Source: CAD feature listing. Evaluate the final solid. Frame: model axes, mm. A direction names the side the tool comes from. Give positions to 0.01 mm unless a question says otherwise; leave off trailing zeros. Order: outer loops, then holes, each group sorted by start corner. A loop starts at its lowest first (then second) coordinate and runs counter-clockwise, first axis right, second up. Notation, with made-up numbers: M 82,61.5 L 137,61.5 A20 ccw 137,84.5 Z; hole C 67,-6 d1. An arc over 180 degrees is marked long. Answer in a Markdown table with one row per item. Add a question column.
(1) Section query D-D, the plane z = 8. Return loops of the section in (x, y), plus the area to 3 significant figures.
(2) Set-up query: faces 1 (the face through (-1, 6, -4)), 2 (the face through (0.423, 7.222, -8.514)), 3 (the face through (3, 6, -9.5)), 4 (the face through (5.752, 5.387, -0.099)), 5 (the face through (2, 0, 3)). Return all of +Z, -Z, +X, -X, +Y, -Y with unobstructed straight access to the full face (end or side cutting, diameter ignored); none if empty.
(3) Section query A-A, the plane z = 0. Return loops of the section in (x, y).
(4) Pin query (flat end, axial travel): P1, Ø3, axis at x = -5.5, y = 6, coming from the +Z side; P2, Ø2, axis at x = -8, z = 0.5, coming from the +Y side; P3, Ø3, axis at y = 5.5, z = -5.5, coming from the +X side. Return the tip coordinate at first contact, or that it passes through.
(5) Material intervals for line 1 along X through (y, z) = (7, -1.25); line 2 along Z through (x, y) = (1.75, 2.75); line 3 along Y through (x, z) = (8, 1.5), sorted ascending.
(6) Section query C-C, the plane x = 0. Return loops of the section in (y, z).
(7) Mould query, pull axis Z, two halves, no side actions, for faces 6 (the face through (-0.29, 5.39, 5.77)), 7 (the face through (2, 8, 3)), 8 (the face through (-0.406, 3.944, 11.243)). Classes: pulls with the +Z half, pulls with the -Z half, needs draft (parallel to the pull), parting line crosses it, or undercut.
(8) Section query B-B, the plane y = 4. Return loops of the section in (x, z).
from build123d import *

# Parameters (mm, degrees)
BOSS_EXTRU_1_DEPTH                              = 8
SKETCH1_R                                       = 3.2
CUT_EXTRUDE1_DEPTH                              = 18.808003819
ESQUISSE7_W                                     = 7
ESQUISSE7_H                                     = 3.5
ENL_V_MAT_EXTRU_2_DEPTH                         = 18.808003819
CHAMBRAGE_POUR_VIS_T_TE_CYLINDRIQUE_D           = 2.5
CHAMBRAGE_POUR_VIS_T_TE_CYLINDRIQUE_CBORE_D     = 4.5
CHAMBRAGE_POUR_VIS_T_TE_CYLINDRIQUE_CBORE_DEPTH = 5.3
CBORE_FOR_M5_HEX_HEAD_BOLT1_D                   = 4
CBORE_FOR_M5_HEX_HEAD_BOLT1_DEPTH               = 9.499
CBORE_FOR_M5_HEX_HEAD_BOLT1_CBORE_D             = 6.5
CBORE_FOR_M5_HEX_HEAD_BOLT1_CBORE_DEPTH         = 2
CBORE_FOR_M5_HEX_HEAD_BOLT1_TIP                 = 1.201721238


with BuildPart() as part:
    # Esquisse1 → Boss.-Extru.1 (new body)
    with BuildSketch(Plane(origin=(0, 0, 0), x_dir=(1, 0, 0), z_dir=(0, 1, 0))):
        with BuildLine():
            Line((6.025985397, 9.5), (-6.025985397, 9.5))
            ThreePointArc((-6.025985397, 9.5), (0, -11.25), (6.025985397, 9.5))
        make_face()
    extrude(amount=BOSS_EXTRU_1_DEPTH)

    # Sketch1 → Cut-Extrude1 (cut, through all)
    with BuildSketch(Plane(origin=(0, 8, 0), x_dir=(1, 0, 0), z_dir=(0, 1, 0))):
        with Locations(Location((0, 0, 0), (0, 0, 270))):
            Circle(SKETCH1_R)
    extrude(amount=-CUT_EXTRUDE1_DEPTH, mode=Mode.SUBTRACT)

    # Esquisse7 → Enlèv. mat.-Extru.2 (cut, through all)
    with BuildSketch(Plane(origin=(0, 8, 0), x_dir=(1, 0, 0), z_dir=(0, 1, 0))):
        with Locations((0, 5.75)):
            Rectangle(ESQUISSE7_W, ESQUISSE7_H)
    extrude(amount=-ENL_V_MAT_EXTRU_2_DEPTH, mode=Mode.SUBTRACT)

    # Chambrage pour vis à tête cylindrique à 6 pans creux (ou vis CHC) M21 (through all)
    with Locations(Plane(origin=(0, 8, 0), x_dir=(1, 0, 0), z_dir=(0, 1, 0))):
        with Locations((-8, 0), (0, -8), (8, 0)):
            CounterBoreHole(CHAMBRAGE_POUR_VIS_T_TE_CYLINDRIQUE_D / 2, CHAMBRAGE_POUR_VIS_T_TE_CYLINDRIQUE_CBORE_D / 2, CHAMBRAGE_POUR_VIS_T_TE_CYLINDRIQUE_CBORE_DEPTH)

    # CBORE for M5 Hex Head Bolt1
    with Locations(Plane(origin=(0, 0, -9.5), x_dir=(-1, 0, 0), z_dir=(0, 0, -1))):
        with Locations((0, 4)):
            CounterBoreHole(CBORE_FOR_M5_HEX_HEAD_BOLT1_D / 2, CBORE_FOR_M5_HEX_HEAD_BOLT1_CBORE_D / 2, CBORE_FOR_M5_HEX_HEAD_BOLT1_CBORE_DEPTH, depth=CBORE_FOR_M5_HEX_HEAD_BOLT1_DEPTH)
            with Locations((0, 0, -(CBORE_FOR_M5_HEX_HEAD_BOLT1_DEPTH + CBORE_FOR_M5_HEX_HEAD_BOLT1_TIP / 2))):  # 118° drill point
                Cone(0, CBORE_FOR_M5_HEX_HEAD_BOLT1_D / 2, CBORE_FOR_M5_HEX_HEAD_BOLT1_TIP, mode=Mode.SUBTRACT)


solid = part.part
Values follow:
| question | item | result |
|---|---|---|
| 1 | outline | M -7.91,0 L -1.25,0 L -1.25,2.7 L -2.25,2.7 L -2.25,8 L -7.91,8 Z; M 1.25,0 L 7.91,0 L 7.91,8 L 2.25,8 L 2.25,2.7 L 1.25,2.7 Z |
| 1 | area | 96.0 mm² |
| 2 | face 1 | +Y, -Y |
| 2 | face 2 | -Z |
| 2 | face 3 | -Z, +X, -X, +Y, -Y |
| 2 | face 4 | +Y |
| 2 | face 5 | +Z, -Z, +X, -X, -Y |
| 3 | outline | M -11.25,0 L -9.25,0 L -9.25,2.7 L -10.25,2.7 L -10.25,8 L -11.25,8 Z; M -6.75,0 L -3.2,0 L -3.2,8 L -5.75,8 L -5.75,2.7 L -6.75,2.7 Z; M 3.2,0 L 6.75,0 L 6.75,2.7 L 5.75,2.7 L 5.75,8 L 3.2,8 Z; M 9.25,0 L 11.25,0 L 11.25,8 L 10.25,8 L 10.25,2.7 L 9.25,2.7 Z |
| 4 | P1 | stops at z = 10.51 |
| 4 | P2 | stops at y = 2.7 |
| 4 | P3 | stops at x = 10.51 |
| 5 | line 1 | x = -11.18 to -9.87, -6.13 to -2.95, 2.95 to 6.13, 9.87 to 11.18 |
| 5 | line 2 | z = -4 to -2.68, 2.68 to 6.59, 9.41 to 11.11 |
| 5 | line 3 | y = 0 to 2.7 |
| 6 | outline | M 0,-9.5 L 0.75,-9.5 L 0.75,-7.5 L 0,-7.5 Z; M 0,-4 L 2,-4 L 2,-3.2 L 0,-3.2 Z; M 0,3.2 L 8,3.2 L 8,5.75 L 2.7,5.75 L 2.7,6.75 L 0,6.75 Z; M 0,9.25 L 2.7,9.25 L 2.7,10.25 L 8,10.25 L 8,11.25 L 0,11.25 Z; M 6,-4 L 8,-4 L 8,-3.2 L 6,-3.2 Z; M 7.25,-9.5 L 8,-9.5 L 8,-7.5 L 7.25,-7.5 Z |
| 7 | face 6 | undercut |
| 7 | face 7 | needs draft |
| 7 | face 8 | parting line crosses it |
| 8 | outline | M -6.03,-9.5 L -3.25,-9.5 L -3.25,-7.5 L -3.5,-7.5 L -3.5,-4 L -2,-4 L -2,-2.5 A3.2 cw long 2,-2.5 L 2,-4 L 3.5,-4 L 3.5,-7.5 L 3.25,-7.5 L 3.25,-9.5 L 6.03,-9.5 A11.25 ccw long Z; hole C -8,0 d4.5; hole C 0,8 d4.5; hole C 8,0 d4.5 |
